Design review of the part built by this model. Coordinates are the model's own, in mm. A direction names the side the tool comes from. Coordinates: 2 decimals unless noted, no trailing zeros. Write each loop counter-clockwise with the first axis right and the second up, starting at its lowest first coordinate (ties: lowest second). Pieces come first, ordered by that corner, then holes. Notation, with made-up numbers: (84, -33) - (95, -33) arc R32 ccw to (95, 6) - close; hole circle Ø10 at (58.25, -32). An arc over 180 degrees is marked (long way). Use a Markdown table: item, result.
from build123d import *

# Parameters (mm, degrees)
BOSS_EXTRUDE1_DEPTH             = 4
CUT_EXTRUDE2_DEPTH              = 10
BOSS_EXTRUDE2_REACH             = 59.846
BOSS_EXTRUDE2_DIRECTION_2_DEPTH = 28
CUT_EXTRUDE3_DEPTH              = 61.022744116
CUT_EXTRUDE3_DEPTH_BACK         = 61.022744116
SKETCH5_R                       = 1.55
BOSS_EXTRUDE3_DEPTH             = 0.5
CUT_EXTRUDE4_DEPTH              = 53.565024349
BOSS_EXTRUDE4_REACH             = 61.205
BOSS_EXTRUDE4_DIRECTION_2_DEPTH = 28
BOSS_EXTRUDE5_DEPTH             = 0.5


with BuildPart() as part:
    # Sketch1 → Boss-Extrude1 (new, symmetric)
    with BuildSketch(Plane(origin=(0, 0, 0), x_dir=(0, 0, -1), z_dir=(0, 1, 0))):
        Polygon((0, 0), (35, 0), (35, 10), (25, 10), (25, 6), (9.694351386, 6), (5.918748122, 11.392120275), (0, 7.247768223), align=None)
    extrude(amount=BOSS_EXTRUDE1_DEPTH, both=True)

    # Sketch4 → Cut-Extrude2 (cut)
    with BuildSketch(Plane(origin=(0, 0, -35), x_dir=(-1, 0, 0), z_dir=(0, 0, -1))):
        Polygon((10, 4), (7.856406461, 4), (10, -4), align=None)
    extrude(amount=-CUT_EXTRUDE2_DEPTH, mode=Mode.SUBTRACT)

    # Boss-Extrude2: up to this plane
    boss_extrude2_end = Plane(origin=(0, 4, 0), z_dir=(0, 1, 0))
    # Sketch2 → Boss-Extrude2 (add, up to the surface)
    with BuildSketch(Plane(origin=(2.479828187, -7.343959884, 20), x_dir=(-0.96592582628907, 0.25881904510251447, 0), z_dir=(0.25881904510251447, 0.96592582628907, 0)), mode=Mode.PRIVATE) as boss_extrude2_sk1:
        with BuildLine():
            Line((25.037543411, -49), (33.54403058, -49))
            Line((33.54403058, -49), (33.54403058, -47))
            Line((33.54403058, -47), (26.54403058, -47))
            ThreePointArc((26.54403058, -47), (10.920068858, -50), (26.54403058, -53))
            Line((26.54403058, -53), (33.54403058, -53))
            Line((33.54403058, -53), (33.54403058, -51))
            Line((33.54403058, -51), (25.037543411, -51))
            ThreePointArc((25.037543411, -51), (12.920068858, -50), (25.037543411, -49))
        make_face()
    boss_extrude2_tool1 = split(extrude(boss_extrude2_sk1.sketch, amount=BOSS_EXTRUDE2_REACH, mode=Mode.PRIVATE), bisect_by=boss_extrude2_end, keep=Keep.BOTH, mode=Mode.PRIVATE)
    add(boss_extrude2_tool1.solids().sort_by_distance((-25.812899, 0.237054, -28.72174))[0])

    # Sketch2 → Boss-Extrude2 direction 2 (add)
    with BuildSketch(Plane(origin=(2.479828187, -7.343959884, 20), x_dir=(-0.96592582628907, 0.25881904510251447, 0), z_dir=(0.25881904510251447, 0.96592582628907, 0))):
        with BuildLine():
            Line((25.037543411, -49), (33.54403058, -49))
            Line((33.54403058, -49), (33.54403058, -47))
            Line((33.54403058, -47), (26.54403058, -47))
            ThreePointArc((26.54403058, -47), (10.920068858, -50), (26.54403058, -53))
            Line((26.54403058, -53), (33.54403058, -53))
            Line((33.54403058, -53), (33.54403058, -51))
            Line((33.54403058, -51), (25.037543411, -51))
            ThreePointArc((25.037543411, -51), (12.920068858, -50), (25.037543411, -49))
        make_face()
    extrude(amount=-BOSS_EXTRUDE2_DIRECTION_2_DEPTH)

    # Sketch5 → Cut-Extrude3 (cut, two sides: drawn at the far end of the back side and taken through both)
    with BuildSketch(Plane(origin=(0, 0, -35), x_dir=(-1, 0, 0), z_dir=(0, 0, -1)).offset(-CUT_EXTRUDE3_DEPTH_BACK)):
        with Locations((29.206205162, -9.547072736)):
            Circle(SKETCH5_R)
    extrude(amount=CUT_EXTRUDE3_DEPTH + CUT_EXTRUDE3_DEPTH_BACK, mode=Mode.SUBTRACT)

    # Sketch7 → Boss-Extrude3 (add)
    with BuildSketch(Plane(origin=(-8.916806244, -33.277973944, 0), x_dir=(-0.96592582628907, 0.2588190451025145, 0), z_dir=(0.2588190451025145, 0.96592582628907, 0))):
        with BuildLine():
            Line((20.944110699, -29), (19.724981983, -29))
            ThreePointArc((19.724981983, -29), (9.623982082, -30), (19.724981983, -31))
            Line((19.724981983, -31), (20.944110699, -31))
            ThreePointArc((20.944110699, -31), (8.423982082, -30), (20.944110699, -29))
        make_face()
    extrude(amount=BOSS_EXTRUDE3_DEPTH)

    # Sketch8 → Cut-Extrude4 (cut, through all)
    with BuildSketch(Plane(origin=(-6.5287948, 0, -9.32408528), x_dir=(-0.819152044288991, 0, 0.5735764363510473), z_dir=(-0.5735764363510473, 0, -0.819152044288991))):
        Polygon((5.937024156, 4), (5.937024156, -4), (3.793430617, 4), align=None)
    extrude(amount=-CUT_EXTRUDE4_DEPTH, mode=Mode.SUBTRACT)

    # Boss-Extrude4: up to this plane
    boss_extrude4_end = Plane(origin=(0, 4, 0), z_dir=(0, 1, 0))
    # Sketch9 → Boss-Extrude4 (add, up to the surface)
    with BuildSketch(Plane(origin=(-1.144933078, -5.216306847, 0.801690772), x_dir=(-0.5735764363510472, 0, -0.819152044288991), z_dir=(0.21201214989664938, 0.96592582628907, -0.14845250554968126)), mode=Mode.PRIVATE) as boss_extrude4_sk1:
        with BuildLine():
            Line((6.769877721, 16.816923337), (6.769877721, 25.323410506))
            Line((6.769877721, 25.323410506), (4.769877721, 25.323410506))
            Line((4.769877721, 25.323410506), (4.769877721, 18.323410506))
            ThreePointArc((4.769877721, 18.323410506), (7.769877721, 2.699448783), (10.769877721, 18.323410506))
            Line((10.769877721, 18.323410506), (10.769877721, 25.323410506))
            Line((10.769877721, 25.323410506), (8.769877721, 25.323410506))
            Line((8.769877721, 25.323410506), (8.769877721, 16.816923337))
            ThreePointArc((8.769877721, 16.816923337), (7.769877721, 4.699448783), (6.769877721, 16.816923337))
        make_face()
    boss_extrude4_tool1 = split(extrude(boss_extrude4_sk1.sketch, amount=BOSS_EXTRUDE4_REACH, mode=Mode.PRIVATE), bisect_by=boss_extrude4_end, keep=Keep.BOTH, mode=Mode.PRIVATE)
    add(boss_extrude4_tool1.solids().sort_by_distance((-21.539934, 0.237054, 7.157621))[0])

    # Sketch9 → Boss-Extrude4 direction 2 (add)
    with BuildSketch(Plane(origin=(-1.144933078, -5.216306847, 0.801690772), x_dir=(-0.5735764363510472, 0, -0.819152044288991), z_dir=(0.21201214989664938, 0.96592582628907, -0.14845250554968126))):
        with BuildLine():
            Line((6.769877721, 16.816923337), (6.769877721, 25.323410506))
            Line((6.769877721, 25.323410506), (4.769877721, 25.323410506))
            Line((4.769877721, 25.323410506), (4.769877721, 18.323410506))
            ThreePointArc((4.769877721, 18.323410506), (7.769877721, 2.699448783), (10.769877721, 18.323410506))
            Line((10.769877721, 18.323410506), (10.769877721, 25.323410506))
            Line((10.769877721, 25.323410506), (8.769877721, 25.323410506))
            Line((8.769877721, 25.323410506), (8.769877721, 16.816923337))
            ThreePointArc((8.769877721, 16.816923337), (7.769877721, 4.699448783), (6.769877721, 16.816923337))
        make_face()
    extrude(amount=-BOSS_EXTRUDE4_DIRECTION_2_DEPTH)

    # Sketch10 → Boss-Extrude5 (add)
    with BuildSketch(Plane(origin=(-7.081273275, -32.262229983, 4.958360927), x_dir=(0.9766546875566917, -0.2147970934280116, -0.0027982009254068387), z_dir=(-0.21201214989664938, -0.96592582628907, 0.14845250554968126))):
        with BuildLine():
            Line((-16.465765356, 2.911480582), (-17.901629513, 3.876715105))
            ThreePointArc((-17.901629513, 3.876715105), (-8.068915493, -3.938101309), (-19.017417439, 2.216890625))
            Line((-19.017417439, 2.216890625), (-17.581553282, 1.251656102))
            ThreePointArc((-17.581553282, 1.251656102), (-9.479766301, -2.989681571), (-16.465765356, 2.911480582))
        make_face()
    extrude(amount=-BOSS_EXTRUDE5_DEPTH)


solid = part.part
(1) For pin 1 (5 mm diameter, centred on x = -32, y = -15.5, fed in from +Z); pin 2 (1 mm diameter, centred on x = -22.5, z = 8.5, fed in from -Y); pin 3 (3 mm diameter, centred on x = -7.5, y = 2, fed in from +Z), all flat-tipped, find the tip position at first contact; note any pin that passes through.
Determined:
| item | result |
|---|---|
| pin 1 | z = 10.52 |
| pin 2 | y = -28.42 |
| pin 3 | z = 6.68 |
(2) Take a section at A-A on z = -32. Write out the cut boundary in (x, y).
Determined:
| item | result |
|---|---|
| outline | (-37.17, -25.71) - (-27.67, -28.25) - (-27.54, -27.77) - (-28.58, -27.49) - (-20.14, 4) - (-29.21, 4) - close; (-18.61, -30.68) - (-15.56, -31.5) - (-8.19, -4) - (0, -4) - (0, 4) - (-8.21, 4) - (-17.44, -30.48) - (-18.48, -30.2) - close; hole circle Ø3.1 at (-29.21, -9.55) |
(3) For L1, parallel to Z at x = -23.5, y = -26; L2, parallel to Z at x = -25.5, y = -23; L3, parallel to Z at x = -15, y = -28, list the stretches that pass through material, from the lowest coordinate up. Write a range as from..to.
Determined:
| item | result |
|---|---|
| L1 | -38..-35.97, -24.03..-22, -2.9..-0.41, 8.76..11.25 |
| L2 | -37.07..-34.64, -25.36..-22.93, -0.83..7.15, 9.59..12.03 |
| L3 | -33.1..-26.9, -2.51..0.21, 8.19..10.9 |
(4) Take a section at B-B on z = -23. Write out the cut boundary in (x, y), and give its area (3 significant figures).
Determined:
| item | result |
|---|---|
| outline | (-27.08, -28.41) - (-19.2, -30.52) - (-9.95, 4) - (-18.39, 4) - close; (-6, -4) - (0, -4) - (0, 4) - (-6, 4) - close |
| area | 330 mm2 |
(5) Draft analysis for pull direction Y (two halves, no side actions). For faces 1 (the flat face through (-33.132, -10.646, -32.014)), 2 (the flat face through (-18.229, -30.265, -28.164)), 3 (the flat face through (-28, -11, -33)), state which applies: +Y half, -Y half, draft (parallel to the pull), parting line (faces both ways), or undercut.
Determined:
| item | result |
|---|---|
| face 1 | +Y half |
| face 2 | undercut |
| face 3 | draft |
(6) Machinability: for faces 4 (the flat face through (-2, 0, 0)), 5 (the flat face through (-6, 0, -17)), 6 (the flat face through (-23.6, -10.6, 10.7)), 7 (the flat face through (-28.517, -28.026, -28.087)), which of the approach directions +Z, -Z, +X, -X, +Y, -Y give a long, thin tool a straight path to every point of the face, cutting with its end or side? Answer none if there is none.
Determined:
| item | result |
|---|---|
| face 4 | +Z, +X, -Y |
| face 5 | +Y, -Y |
| face 6 | +Z, +Y |
| face 7 | -Z, -X, -Y |
(7) Take a section at C-C on x = -16.5. State how many separate pieces and enclosed holes the cut face has, and give its area (3 significant figures).
Determined:
| item | result |
|---|---|
| separate pieces | 3 |
| enclosed holes | 0 |
| area | 328 mm2 |
